```python
from build123d import *

# Parameters (mm, degrees)
SKETCH5_R             = 0.729
BOSS_EXTRUDE1_DEPTH   = 5.2
BOSS_EXTRUDE1_2_DEPTH = 5.2
BOSS_EXTRUDE1_3_DEPTH = 5.2
SKETCH6_W             = 9.8
SKETCH6_H             = 10
BOSS_EXTRUDE2_DEPTH   = 11.3
SKETCH8_R             = 4.15
BOSS_EXTRUDE3_DEPTH   = 9.4
SKETCH9_R             = 1.5
CUT_EXTRUDE1_DEPTH    = 9.4
FILLET1_R             = 1
FILLET2_R             = 0.5
SKETCH10_W            = 1.469693846
SKETCH10_H            = 1.5
SKETCH10_W_2          = 1.486314294
SKETCH10_H_2          = 1.483532886
BOSS_EXTRUDE4_DEPTH   = 1.5


with BuildPart() as part:
    # Sketch5 → Boss-Extrude1 (new body)
    with BuildSketch(Plane.XY):
        with Locations((44.56, 20.21)):
            Circle(SKETCH5_R)
    extrude(amount=BOSS_EXTRUDE1_DEPTH)



with BuildPart() as body_2:
    # Sketch5 → Boss-Extrude1 2 (new body)
    with BuildSketch(Plane.XY):
        with Locations((44.56, 12.81)):
            Circle(SKETCH5_R)
    extrude(amount=BOSS_EXTRUDE1_2_DEPTH)


with BuildPart() as body_3:
    # Sketch5 → Boss-Extrude1 3 (new body)
    with BuildSketch(Plane.XY):
        with Locations((48.26, 16.51)):
            Circle(SKETCH5_R)
    extrude(amount=BOSS_EXTRUDE1_3_DEPTH)


with BuildPart() as part_1:
    add(part.part)

    add(body_2.part)  # Boss-Extrude2 merges body 2

    add(body_3.part)  # Boss-Extrude2 merges body 3
    # Sketch6 → Boss-Extrude2 (add)
    with BuildSketch(Plane.XY):
        with Locations((47.36, 16.51)):
            Rectangle(SKETCH6_W, SKETCH6_H)
    extrude(amount=-BOSS_EXTRUDE2_DEPTH)

    # Sketch8 → Boss-Extrude3 (add)
    with BuildSketch(Plane(origin=(52.26, 0, 0), x_dir=(0, 0, -1), z_dir=(1, 0, 0))):
        with Locations((5.65, 16.51)):
            Circle(SKETCH8_R)
    extrude(amount=BOSS_EXTRUDE3_DEPTH)

    # Sketch9 → Cut-Extrude1 (cut)
    with BuildSketch(Plane(origin=(61.66, 0, 0), x_dir=(0, 0, -1), z_dir=(1, 0, 0))):
        with Locations((5.65, 16.51)):
            Circle(SKETCH9_R)
    extrude(amount=-CUT_EXTRUDE1_DEPTH, mode=Mode.SUBTRACT)

    # Fillet1
    fillet1_edges = [part_1.edges().sort_by_distance(p)[0] for p in [
        (61.66, 16.51, -1.5),
    ]]
    fillet(fillet1_edges, radius=FILLET1_R)

    # Fillet2
    fillet2_edges = [part_1.edges().sort_by_distance(p)[0] for p in [
        (61.66, 16.51, -4.15),
    ]]
    fillet(fillet2_edges, radius=FILLET2_R)

    # Sketch10 → Boss-Extrude4 (add)
    with BuildSketch(Plane.XY):
        with Locations((51.36, 20.76)):
            Rectangle(SKETCH10_W, SKETCH10_H)
        with Locations((51.36, 12.26)):
            Rectangle(SKETCH10_W_2, SKETCH10_H_2)
    extrude(amount=BOSS_EXTRUDE4_DEPTH)


solid = part_1.part
```
Verification items for the finished model (mm, model axes). A direction names the side the tool comes from. Round coordinates to 2 decimals unless told otherwise and drop trailing zeros. Write each loop counter-clockwise with the first axis right and the second up, starting at its lowest first coordinate (ties: lowest second). Pieces come first, ordered by that corner, then holes. Notation, with made-up numbers: (32, 41.5) -> (83, 41.5) arc R28 ccw to (83, 71.5) -> close; hole circle Ø3 at (46, 66.5). An arc over 180 degrees is marked (long way). Write each question's results on one line, items separated by ' | '.
Q1. Access from +Z, -Z, +X, -X, +Y, -Y to the whole of each face (thin tool, end or side, straight path). Record for faces 4 (the face through (51, 20.01, 1)), 5 (the face through (56.4, 12.46, -4.75)), 6 (the face through (52.103, 12, 1)).
Derived:
face 4: +Z, +X | face 5: +X | face 6: +Z, +X, +Y, -Y
Q2. Sectioned sample at B-B, the plane z = -5.65. Record the boundary of the cut face in (x, y), and give its area (3 significant figures).
Derived:
outline: (42.46, 11.51) -> (52.26, 11.51) -> (52.26, 12.36) -> (60.66, 12.36) arc R1 ccw to (61.66, 13.36) -> (61.66, 14.51) arc R0.5 ccw to (61.16, 15.01) -> (52.26, 15.01) -> (52.26, 18.01) -> (61.16, 18.01) arc R0.5 ccw to (61.66, 18.51) -> (61.66, 19.66) arc R1 ccw to (60.66, 20.66) -> (52.26, 20.66) -> (52.26, 21.51) -> (42.46, 21.51) -> close | area: 147 mm²
Q3. Draft check along X on faces 1 (the face through (52.26, 17, -6)), 2 (the face through (51, 13.002, 1)), 3 (the face through (50.625, 21, 1)). Enter one of: released by +X, released by -X, zero draft, split by the parting line, or undercut.
Derived:
face 1: released by +X | face 2: zero draft | face 3: undercut
Q4. Go/stop test with flat-tipped pins: pin 1 Ø1.6 at (y, z) = (12, 0.5) entering from -X; pin 2 Ø2.5 at (y, z) = (16.51, -5.65) entering from +X; pin 3 Ø2 at (x, y) = (46.5, 16) entering from +Z; pin 4 Ø0.7 at (x, z) = (51, 1) entering from -Y. Record where each tip stops, or that it passes through.
Derived:
pin 1: stops at x = 42.46 | pin 2: stops at x = 52.26 | pin 3: stops at z = 0 | pin 4: stops at y = 11.52
Q5. Thickness scan on probe 1 along Y at (x, z) = (55, -5.65); probe 2 along Z at (x, y) = (53.5, 16); probe 3 along X at (y, z) = (16.25, -5.5). Record the ranges inside material, lowest first.
Derived:
probe 1: y = 12.36 to 15.01, 18.01 to 20.66 | probe 2: z = -9.77 to -7.06, -4.24 to -1.53 | probe 3: x = 42.46 to 52.26
Q6. Sectioned sample at D-D, the plane x = 48.26. Record the boundary of the cut face in (y, z).
Derived:
outline: (11.51, -11.3) -> (21.51, -11.3) -> (21.51, 0) -> (17.24, 0) -> (17.24, 5.2) -> (15.78, 5.2) -> (15.78, 0) -> (11.51, 0) -> close
Q7. Sectioned sample at A-A, the plane x = 44.56. Record the boundary of the cut face in (y, z), and give its area (3 significant figures).
Derived:
outline: (11.51, -11.3) -> (21.51, -11.3) -> (21.51, 0) -> (20.94, 0) -> (20.94, 5.2) -> (19.48, 5.2) -> (19.48, 0) -> (13.54, 0) -> (13.54, 5.2) -> (12.08, 5.2) -> (12.08, 0) -> (11.51, 0) -> close | area: 128 mm²
Q8. Sectioned sample at C-C, the plane x = 58.5. Record the boundary of the cut face in (y, z).
Derived:
outline: circle Ø8.3 at (16.51, -5.65); hole circle Ø3 at (16.51, -5.65)
